Solid Edge part; units mm, degrees
sketch "Sketch1" plane through (0, 0, 0) normal (0, 0, 1) x (1, 0, 0)
  line L0 (85, 5) -> (5, 5)
  arc A0 (0, 0) -> (5, 5) centre (5, 0) cw
  line L1 (0, 0) -> (0, -45)
  arc A1 (0, -45) -> (5, -50) centre (5, -45) ccw
  line L2 (5, -50) -> (85, -50)
  arc A2 (90, -45) -> (85, -50) centre (85, -45) cw
  line L3 (90, -45) -> (90, 0)
  arc A3 (85, 5) -> (90, 0) centre (85, 0) cw
sketch "Sketch2" plane through (0, 0, 0) normal (0, -1, 0) x (1, 0, 0)
  line L0 (-12, 0) -> (-8.5, 0)
  line L1 (-8.5, 11) -> (-8.5, 0)
  line L2 (-8.5, 11) -> (-17, 11)
  line L3 (-23, 11) -> (-17, 11)
  line L4 (-23, 11) -> (-23, 8.8)
  line L5 (-23, 8.8) -> (-27, 8.8)
  line L6 (-27, 8.8) -> (-27, 0)
  line L7 (-27, 0) -> (-25.5, 0)
  line L8 (-25.5, 0) -> (-25.5, 6.5)
  line L9 (-25.5, 6.5) -> (-18.5, 6.5)
  line L10 (-18.5, 6.5) -> (-18.5, 0)
  line L11 (-12, 0) -> (-18.5, 0)
sweep "SweptProtrusion_13" add profiles "Sketch2" path "Sketch1"
Geometry check sheet. Reference: the model listing, model coordinates, mm. A direction names the side the tool comes from. Round coordinates to 2 decimals unless told otherwise and drop trailing zeros. Loops run counter-clockwise (first coordinate to the right, second up) from the corner with the lowest first, then second, coordinate; pieces in that order, holes last. Notation, with made-up numbers: (29, 27.25) -> (57, 27.25) arc R20 cw to (57, 52.25) -> close; hole circle Ø7 at (67.5, 18.25). An arc over 180 degrees is marked (long way). Answer as a JSON object with one key per item and string values. Group by question number.
Item 1: Set-up check for faces 4 (the face through (107.38, 22.87, 4.34)), 5 (the face through (-4.65, -54.44, 5.58)), 6 (the face through (106.8, 21.33, 3.3)), 7 (the face through (-14.58, -65.015, 9.885)), 8 (the face through (107.87, -67.38, 4.34)): record each of +Z, -Z, +X, -X, +Y, -Y from which the full face is reachable in a straight line by a thin tool's end or side.
Item 2: Thickness scan on line 1 along Y through (x, z) = (21.5, 6.25); line 2 along X through (y, z) = (-37.5, 4.75); line 3 along X through (y, z) = (2, 1). Record the ranges inside material, lowest first.
Item 3: Depth check by flat-ended pin: pin 1 Ø1.1 at (x, z) = (60.5, 10) entering from -Y; pin 2 Ø0.7 at (y, z) = (-26.5, 10) entering from -X; pin 3 Ø0.7 at (x, z) = (27, 10) entering from +Y. Enter the tip coordinate at first touch or a pass-through.
Item 4: Cross-section at D-D, the plane y = 18. Record the cut outline in (x, z), plus the area to 3 significant figures.
Item 5: Cross-section at A-A, the plane y = -42. Record the cut outline in (x, z), plus the area to 3 significant figures.
Item 6: Release check for a two-part mould opening along Y. For faces 1 (the face through (104.58, 20.015, 9.885)), 2 (the face through (106.33, -66.8, 3.3)), 3 (the face through (-17.38, -67.87, 4.34)) record: pulls with the +Y half, pulls with the -Y half, needs draft (parallel to the pull), parting line crosses it, or undercut.
Item 7: Cross-section at C-C, the plane z = 2.25. Count the separate pieces of the cut face and the enclosed holes in it, plus the area to 3 significant figures.
Item 8: Cross-section at B-B, the plane x = 39.5. Record the cut outline in (y, z).
Determined:
{
 "1": {"face 4": "+Z, -Z, +X, +Y", "face 5": "+Z, -Z", "face 6": "-Z", "face 7": "+Z, -X, -Y", "face 8": "+Z, -Z, +X, -Y"},
 "2": {"line 1": "y = -77 to -75.5, -68.5 to -58.5, 13.5 to 23.5, 30.5 to 32", "line 2": "x = -27 to -25.5, -18.5 to -8.5, 98.5 to 108.5, 115.5 to 117", "line 3": "x = -26.94 to -25.43, -18.41 to -8.35, 98.35 to 108.41, 115.43 to 116.94"},
 "3": {"pin 1": "stops at y = -73", "pin 2": "stops at x = -23", "pin 3": "stops at y = 28"},
 "4": {"outline": "(-21.46, 0) -> (-19.62, 0) -> (-19.62, 6.5) -> (-10.11, 6.5) -> (-10.11, 0) -> (100.11, 0) -> (100.11, 6.5) -> (109.62, 6.5) -> (109.62, 0) -> (111.46, 0) -> (111.46, 8.8) -> (106.45, 8.8) -> (106.45, 11) -> (-16.45, 11) -> (-16.45, 8.8) -> (-21.46, 8.8) -> close", "area": "1,320 mm²"},
 "5": {"outline": "(-27, 0) -> (-25.5, 0) -> (-25.5, 6.5) -> (-18.5, 6.5) -> (-18.5, 0) -> (-8.5, 0) -> (-8.5, 11) -> (-23, 11) -> (-23, 8.8) -> (-27, 8.8) -> close; (98.5, 0) -> (108.5, 0) -> (108.5, 6.5) -> (115.5, 6.5) -> (115.5, 0) -> (117, 0) -> (117, 8.8) -> (113, 8.8) -> (113, 11) -> (98.5, 11) -> close", "area": "298 mm²"},
 "6": {"face 1": "pulls with the +Y half", "face 2": "undercut", "face 3": "pulls with the -Y half"},
 "7": {"separate pieces": "2", "enclosed holes": "2", "area": "4,330 mm²"},
 "8": {"outline": "(-77, 0) -> (-75.5, 0) -> (-75.5, 6.5) -> (-68.5, 6.5) -> (-68.5, 0) -> (-58.5, 0) -> (-58.5, 11) -> (-73, 11) -> (-73, 8.8) -> (-77, 8.8) -> close; (13.5, 0) -> (23.5, 0) -> (23.5, 6.5) -> (30.5, 6.5) -> (30.5, 0) -> (32, 0) -> (32, 8.8) -> (28, 8.8) -> (28, 11) -> (13.5, 11) -> close"}
}
